```python
from build123d import *

# Parameters (mm, degrees)
ESBO_O2_R                = 2.5
RESSALTO_EXTRUS_O1_DEPTH = 20.3
ESBO_O3_R                = 1.75
CORTE_EXTRUS_O1_DEPTH    = 20.3
ESBO_O4_W                = 10.45
ESBO_O4_H                = 20.3
CORTE_EXTRUS_O3_DEPTH    = 8.5
ESBO_O5_W                = 20.3
ESBO_O5_H                = 10.45
CORTE_EXTRUS_O4_DEPTH    = 8.5
ESBO_O6_W                = 10.45
ESBO_O6_H                = 20.3
CORTE_EXTRUS_O5_DEPTH    = 8.5
ESBO_O7_W                = 20.3
ESBO_O7_H                = 10.45
CORTE_EXTRUS_O6_DEPTH    = 8.5
ESBO_O8_R                = 1.75
CORTE_EXTRUS_O7_DEPTH    = 8
ESBO_O10_R               = 1.75
CORTE_EXTRUS_O8_DEPTH    = 8
ESBO_O9_R                = 1.75
CORTE_EXTRUS_O9_DEPTH    = 8
CORTE_EXTRUS_O10_DEPTH   = 21.3000001
CORTE_EXTRUS_O13_DEPTH   = 21.3000001


with BuildPart() as part:
    # Esboço2 → Ressalto-extrusão1 (new body)
    with BuildSketch(Plane.XY):
        with BuildLine():
            ThreePointArc((43.137997257, 25.280688137), (0, 50), (-43.137997257, 25.280688137))
            ThreePointArc((-43.137997257, 25.280688137), (-41.634338387, 18.617028874), (-34.88523184, 19.672919779))
            ThreePointArc((-34.88523184, 19.672919779), (0, 40.050008404), (34.88523184, 19.672919779))
            ThreePointArc((34.88523184, 19.672919779), (41.634338387, 18.617028874), (43.137997257, 25.280688137))
        make_face()
        with Locations((-38.824197531, 22.752619324)):
            Circle(ESBO_O2_R, mode=Mode.SUBTRACT)
        with Locations((38.824197531, 22.752619324)):
            Circle(ESBO_O2_R, mode=Mode.SUBTRACT)
    extrude(amount=RESSALTO_EXTRUS_O1_DEPTH)

    # Esboço3 → Corte-extrusão1 (cut)
    with BuildSketch(Plane(origin=(15.450849719, 47.552825815, 0), x_dir=(0.951056516, -0.309016994, 0), z_dir=(0.309016994, 0.951056516, 0))):
        with Locations((0, -2.42)):
            Circle(ESBO_O3_R)
    extrude(amount=-CORTE_EXTRUS_O1_DEPTH, mode=Mode.SUBTRACT)

    # Esboço4 → Corte-extrusão3 (cut)
    with BuildSketch(Plane(origin=(15.450849719, 47.552825815, 0), x_dir=(0.951056516, -0.309016994, 0), z_dir=(0.309016994, 0.951056516, 0))):
        with Locations((0, -10.15)):
            Rectangle(ESBO_O4_W, ESBO_O4_H)
    extrude(amount=-CORTE_EXTRUS_O3_DEPTH, mode=Mode.SUBTRACT)

    # Esboço5 → Corte-extrusão4 (cut)
    with BuildSketch(Plane(origin=(37.157241274, 33.456530318, 0), x_dir=(0, 0, -1), z_dir=(0.743144825, 0.669130606, 0))):
        with Locations((-10.15, 0)):
            Rectangle(ESBO_O5_W, ESBO_O5_H)
    extrude(amount=-CORTE_EXTRUS_O4_DEPTH, mode=Mode.SUBTRACT)

    # Esboço6 → Corte-extrusão5 (cut)
    with BuildSketch(Plane(origin=(-15.450849719, 47.552825815, 0), x_dir=(0.951056516, 0.309016994, 0), z_dir=(-0.309016994, 0.951056516, 0))):
        with Locations((0, -10.15)):
            Rectangle(ESBO_O6_W, ESBO_O6_H)
    extrude(amount=-CORTE_EXTRUS_O5_DEPTH, mode=Mode.SUBTRACT)

    # Esboço7 → Corte-extrusão6 (cut)
    with BuildSketch(Plane(origin=(-37.157241274, 33.456530318, 0), x_dir=(0, 0, 1), z_dir=(-0.743144825, 0.669130606, 0))):
        with Locations((10.15, 0)):
            Rectangle(ESBO_O7_W, ESBO_O7_H)
    extrude(amount=-CORTE_EXTRUS_O6_DEPTH, mode=Mode.SUBTRACT)

    # Esboço8 → Corte-extrusão7 (cut)
    with BuildSketch(Plane(origin=(30.840510257, 27.768920164, 0), x_dir=(0, 0, -1), z_dir=(0.743144825, 0.669130606, 0))):
        with Locations((-2.42, 0)):
            Circle(ESBO_O8_R)
    extrude(amount=-CORTE_EXTRUS_O7_DEPTH, mode=Mode.SUBTRACT)

    # Esboço10 → Corte-extrusão8 (cut)
    with BuildSketch(Plane(origin=(-30.840510257, 27.768920164, 0), x_dir=(0, 0, 1), z_dir=(-0.743144825, 0.669130606, 0))):
        with Locations((2.42, 0)):
            Circle(ESBO_O10_R)
    extrude(amount=-CORTE_EXTRUS_O8_DEPTH, mode=Mode.SUBTRACT)

    # Esboço9 → Corte-extrusão9 (cut)
    with BuildSketch(Plane(origin=(-12.824205267, 39.468845426, 0), x_dir=(0.951056516, 0.309016994, 0), z_dir=(-0.309016994, 0.951056516, 0))):
        with Locations((0, -2.42)):
            Circle(ESBO_O9_R)
    extrude(amount=-CORTE_EXTRUS_O9_DEPTH, mode=Mode.SUBTRACT)

    # Esboço11 → Corte-extrusão10 (cut, through all)
    with BuildSketch(Plane.XY.offset(20.3)):
        with BuildLine():
            Line((-40.450008581, 29.390420306), (-38.593336029, 27.718664832))
            ThreePointArc((-38.593336029, 27.718664832), (-41.446519528, 26.976164323), (-43.377460924, 24.74828901))
            Line((-43.377460924, 24.74828901), (-42.327289397, 29.390420306))
            Line((-42.327289397, 29.390420306), (-40.450008581, 29.390420306))
        make_face()
        with BuildLine():
            Line((38.629484885, 27.751213408), (40.450008581, 29.390420306))
            Line((40.450008581, 29.390420306), (42.795606827, 28.974236974))
            Line((42.795606827, 28.974236974), (42.969901633, 25.552082367))
            ThreePointArc((42.969901633, 25.552082367), (41.08508844, 27.214931295), (38.629484885, 27.751213408))
        make_face()
    extrude(amount=-CORTE_EXTRUS_O10_DEPTH, mode=Mode.SUBTRACT)

    # Esboço13 → Corte-extrusão13 (cut, through all)
    with BuildSketch(Plane.XY.offset(20.3)):
        with BuildLine():
            Line((-43.591003867, 44.387154562), (-0.084802266, 65.050582409))
            Line((-0.084802266, 65.050582409), (44.470714032, 40.916344415))
            Line((44.470714032, 40.916344415), (33.115675704, 30.468869731))
            ThreePointArc((33.115675704, 30.468869731), (-0.45988999, 44.997649952), (-33.731495865, 29.785670828))
            Line((-33.731495865, 29.785670828), (-43.591003867, 44.387154562))
        make_face()
    extrude(amount=-CORTE_EXTRUS_O13_DEPTH, mode=Mode.SUBTRACT)


solid = part.part
```
Geometry: final body of the model. Coordinates: model frame, mm. A direction names the side the tool comes from. Round coordinates to 2 decimals unless told otherwise and drop trailing zeros. Write each loop counter-clockwise with the first axis right and the second up, starting at its lowest first coordinate (ties: lowest second). Pieces come first, ordered by that corner, then holes. Notation, with made-up numbers: M -8.75,84.5 L 33.25,84.5 A13 ccw 33.25,98.5 Z; hole C 0,69.25 d8. An arc over 180 degrees is marked long. Answer in a Markdown table with one row per item. Add a question column.
(1) Ray query, L1, parallel to X at y = 22, z = 7; L2, parallel to X at y = 22.5, z = 7.5; L3, parallel to X at y = 35.75, z = 5.5. Return the intervals inside material, ascending.
(2) Contact query for flat-ended pins moving along their axis: pin 1 (12 mm diameter, centred on y = 29, z = 6.5, fed in from -X); pin 2 (2 mm diameter, centred on x = -31.5, z = 12, fed in from +Y); pin 3 (1 mm diameter, centred on x = -8.5, z = 12.5, fed in from -Y). Output: stop coordinate, or through.
(3) Draft query along X for faces 1 (the face through (-24.43, 37.79, 10.29)), 2 (the face through (30.792, 27.823, 10.292)), 3 (the face through (24.586, 37.69, 10.292)). Return one class per face: pulls with the +X half, pulls with the -X half, needs draft (parallel to the pull), parting line crosses it, or undercut.
(4) Cut plane B-B, the plane z = 7.75. Give the number of separate pieces and of enclosed holes in the cut face, then the cut area to 3 significant figures.
(5) Cut plane D-D, the plane x = 20. Return the cut outline in (y, z).
(6) Reachability of faces 4 (the face through (10.935, 39.311, 2.343)), 5 (the face through (8.356, 42.624, 10.292)), 6 (the face through (-30.792, 27.823, 10.008)), 7 (the face through (-18.294, 39.395, 10.292)) from +Z, -Z, +X, -X, +Y, -Y: full face, straight path, thin tool, end or side. Return the list, or none.
(7) Cut plane A-A, the plane y = 32.5. Return the cut outline in (x, z).
(8) Cut plane C-C, the plane x = -33. Return the cut outline in (y, z), then the cut area to 3 significant figures.
Established:
| question | item | result |
|---|---|---|
| 1 | L1 | -43.77 to -41.21, -36.44 to -33.47, 33.47 to 36.44, 41.21 to 43.77 |
| 1 | L2 | -43.82 to -41.31, -36.34 to -33.13, 33.13 to 36.34, 41.31 to 43.82 |
| 1 | L3 | -27.33 to -18.05, 18.05 to 27.33 |
| 2 | pin 1 | x = -43.82 |
| 2 | pin 2 | y = 28.15 |
| 2 | pin 3 | y = 39.03 |
| 3 | face 1 | pulls with the -X half |
| 3 | face 2 | undercut |
| 3 | face 3 | pulls with the +X half |
| 4 | separate pieces | 1 |
| 4 | enclosed holes | 2 |
| 4 | area | 372 mm² |
| 5 | outline | M 34.7,0 L 40.31,0 L 40.31,20.3 L 34.7,20.3 Z |
| 6 | face 4 | none |
| 6 | face 5 | +Z, -Z, +X |
| 6 | face 6 | +Z, -Z |
| 6 | face 7 | +Z, -Z, +Y |
| 7 | outline | M -28.29,0 L -23.4,0 L -23.4,20.3 L -28.29,20.3 Z; M 23.4,0 L 28.29,0 L 28.29,20.3 L 23.4,20.3 Z |
| 8 | outline | M 22.69,0 L 25.37,0 L 25.37,20.3 L 22.69,20.3 Z |
| 8 | area | 54.3 mm² |
